from build123d import *

# Parameters (mm, degrees)
F0_R     = 3.175
F1_DEPTH = 3.175
F2_R     = 8.1915


with BuildPart() as f1:
    # F0 (on Top) → F1 (new body)
    with BuildSketch(Plane.XY):
        with BuildLine():
            ThreePointArc((-15.5081209619, -65.37452), (-10.36179917, -75.1896860078), (0, -79.121))
            ThreePointArc((0, -79.121), (10.36179917, -75.1896860078), (15.5081209619, -65.37452))
            ThreePointArc((15.5081209619, -65.37452), (15.5927547044, -64.4389577876), (15.621, -63.5))
            ThreePointArc((15.621, -63.5), (15.602952529, -62.7493247194), (15.5488518178, -62.000384))
            ThreePointArc((15.5488518178, -62.000384), (0, -47.879), (-15.5488518178, -62.000384))
            ThreePointArc((-15.5488518178, -62.000384), (-15.6198619711, -63.6885550396), (-15.5081209619, -65.37452))
        make_face()
        with BuildLine():
            ThreePointArc((0, -66.675), (-2.2450640303, -61.2549359697), (3.175, -63.5))
            ThreePointArc((3.175, -63.5), (2.2450640303, -65.7450640303), (0, -66.675))
        make_face(mode=Mode.SUBTRACT)
        with BuildLine():
            ThreePointArc((15.5081209619, -65.37452), (10.36179917, -75.1896860078), (0, -79.121))
            Line((0, -79.121), (0, -100.0125))
            Line((0, -100.0125), (0, -104.775))
            ThreePointArc((0, -104.775), (6.7351920908, -107.5648079092), (9.525, -114.3))
            ThreePointArc((9.525, -114.3), (9.5077772588, -114.8725352363), (9.4561713182, -115.443))
            Line((9.4561713182, -115.443), (15.5081209619, -65.37452))
        make_face()
        with BuildLine():
            ThreePointArc((6.35, -100.0125), (3.175, -103.1875), (0, -100.0125))
            ThreePointArc((0, -100.0125), (3.175, -96.8375), (6.35, -100.0125))
        make_face(mode=Mode.SUBTRACT)
        with BuildLine():
            Line((0, -100.0125), (0, -79.121))
            ThreePointArc((0, -79.121), (-10.36179917, -75.1896860078), (-15.5081209619, -65.37452))
            Line((-15.5081209619, -65.37452), (-9.4561713182, -115.443))
            ThreePointArc((-9.4561713182, -115.443), (-7.1278573218, -107.9818297744), (0, -104.775))
            Line((0, -104.775), (0, -100.0125))
        make_face()
        with BuildLine():
            ThreePointArc((9.525, -114.3), (6.7351920908, -107.5648079092), (0, -104.775))
            ThreePointArc((0, -104.775), (-7.1278573218, -107.9818297744), (-9.4561713182, -115.443))
            ThreePointArc((-9.4561713182, -115.443), (0, -123.825), (9.4561713182, -115.443))
            ThreePointArc((9.4561713182, -115.443), (9.5077772588, -114.8725352363), (9.525, -114.3))
        make_face()
        with BuildLine():
            ThreePointArc((3.175, -114.3), (-2.2450640303, -116.5450640303), (0, -111.125))
            ThreePointArc((0, -111.125), (2.2450640303, -112.0549359697), (3.175, -114.3))
        make_face(mode=Mode.SUBTRACT)
        with BuildLine():
            Line((-10.4524001899, -9.157542126), (-15.5488518178, -62.000384))
            ThreePointArc((-15.5488518178, -62.000384), (0, -47.879), (15.5488518178, -62.000384))
            Line((15.5488518178, -62.000384), (9.481007206, 0.9144))
            ThreePointArc((9.481007206, 0.9144), (9.5139954445, 0.4577288296), (9.525, 0))
            ThreePointArc((9.525, 0), (6.6138273175, -6.8544083052), (-0.3401786278, -9.5189234423))
            Line((-0.3401786278, -9.5189234423), (-10.4524001899, -9.157542126))
        make_face()
        with BuildLine():
            Line((-9.481007206, 0.9144), (-10.4524001899, -9.157542126))
            Line((-10.4524001899, -9.157542126), (-0.3401786278, -9.5189234423))
            ThreePointArc((-0.3401786278, -9.5189234423), (-7.164320087, -6.2767939819), (-9.481007206, 0.9144))
        make_face()
        with BuildLine():
            Line((-44.7334821429, -7.9324362036), (-10.4524001899, -9.157542126))
            Line((-10.4524001899, -9.157542126), (-9.481007206, 0.9144))
            ThreePointArc((-9.481007206, 0.9144), (-6.5286581491, 6.9355784022), (-0.3401783155, 9.5189234535))
            Line((-0.3401783155, 9.5189234535), (-44.7334821429, 7.9324362036))
            ThreePointArc((-44.7334821429, 7.9324362036), (-38.9384772185, 5.7120069047), (-36.5125, 0))
            ThreePointArc((-36.5125, 0), (-38.9384772185, -5.7120069047), (-44.7334821429, -7.9324362036))
        make_face()
        with BuildLine():
            ThreePointArc((9.525, 0), (9.5139954445, 0.4577288296), (9.481007206, 0.9144))
            ThreePointArc((9.481007206, 0.9144), (6.2767940994, 7.164319984), (-0.3401783155, 9.5189234535))
            ThreePointArc((-0.3401783155, 9.5189234535), (-6.5286581491, 6.9355784022), (-9.481007206, 0.9144))
            ThreePointArc((-9.481007206, 0.9144), (-7.164320087, -6.2767939819), (-0.3401786278, -9.5189234423))
            ThreePointArc((-0.3401786278, -9.5189234423), (6.6138273175, -6.8544083052), (9.525, 0))
        make_face()
        Circle(F0_R, mode=Mode.SUBTRACT)
        with BuildLine():
            ThreePointArc((-44.7334821429, 7.9324362036), (-52.3875, 0), (-44.7334821429, -7.9324362036))
            ThreePointArc((-44.7334821429, -7.9324362036), (-38.9384772185, -5.7120069047), (-36.5125, 0))
            ThreePointArc((-36.5125, 0), (-38.9384772185, 5.7120069047), (-44.7334821429, 7.9324362036))
        make_face()
        with Locations((-44.45, 0)):
            Circle(F0_R, mode=Mode.SUBTRACT)
    extrude(amount=F1_DEPTH)

    # F2
    f2_edges = [f1.edges().sort_by_distance(p)[0] for p in [
        (-10.4524, -9.157542, 1.5875),
    ]]
    fillet(f2_edges, radius=F2_R)


solid = f1.part
Can you work these out from the model? Positions are in its coordinate system, mm. A direction names the side the tool comes from. Give positions to 0.01 mm unless a question says otherwise; leave off trailing zeros. Loops run counter-clockwise (first coordinate to the right, second up) from the corner with the lowest first, then second, coordinate; pieces in that order, holes last. Notation, with made-up numbers: (-7, -11.5) - (29, -11.5) arc R19 ccw to (29, 21.5) - close; hole circle Ø1 at (73.5, -6.5). An arc over 180 degrees is marked (long way). One line per item, written item: value.
(1) If we section it at A-A, the plane x = -13.5: List the corners of the cut face in (y, z) for me (3 decimals).
Verdict:
outline: (-81.988, 0) - (-40.757, 0) - (-40.757, 3.175) - (-81.988, 3.175) - close; (-11.394, 0) - (9.049, 0) - (9.049, 3.175) - (-11.394, 3.175) - close
(2) I'm going to push flat-ended pins straight in: pin 1 (4 mm diameter, centred on x = 0, y = -63.5, fed in from +Z); pin 2 (1.5 mm diameter, centred on y = -10, z = 0.5, fed in from +X); pin 3 (7.5 mm diameter, centred on x = 0, y = -114.3, fed in from +Z) (3 decimals); pin 4 (1 mm diameter, centred on y = -37.5, z = 2, fed in from +X). Where does each tip first touch, or does it pass through?
Verdict:
pin 1: through
pin 2: x = 10.61
pin 3: z = 3.175
pin 4: x = 13.23
(3) If we mould it in two halves opening along X, with no side actions, what happens to faces 1 (the face through (12.557, -30.983, 1.565)), 2 (the face through (3.863, -103.112, 1.565)), 3 (the face through (-12.525, -90.058, 1.565)), 4 (the face through (-0.69, -3.1, 1.57))? For each: released by +X, released by -X, zero draft, split by the parting line, or undercut.
Verdict:
face 1: released by +X
face 2: undercut
face 3: released by -X
face 4: undercut
(4) On a 3-axis mill with a long thin cutter (end or side, diameter ignored), from which of +Z, -Z, +X, -X, +Y, -Y can I reach the whole of each face in a straight line? I mean faces 5 (the face through (-41.42, 0.95, 1.57)), 6 (the face through (-13.39, -39.6, 1.57)). Say none if no direction works.
Verdict:
face 5: +Z, -Z
face 6: +Z, -Z, -X
(5) If we section it at D-D, the plane y = -46: List the corners of the cut face in (x, z) for me (3 decimals).
Verdict:
outline: (-14.006, 0) - (14.006, 0) - (14.006, 3.175) - (-14.006, 3.175) - close
(6) I need wall thicknesses on line 1 along Y through (x, z) = (-44.45, 0.7) (3 decimals); line 2 along X through (y, z) = (-63.5, 0.9) (3 decimals); line 3 along Y through (x, z) = (-1.5, 0.7). Which ranges of each line are inside material? Lowest first, please.
Verdict:
line 1: -7.943 to -3.175, 3.175 to 7.943
line 2: -15.621 to -3.175, 3.175 to 15.621
line 3: -123.71 to -117.1, -111.5 to -66.3, -60.7 to -2.8, 2.8 to 9.48
(7) If we section it at C-C, the plane x = -43: List the corners of the cut face in (y, z) for me (3 decimals), plus the area to 3 significant figures.
Verdict:
outline: (-7.994, 0) - (-2.825, 0) - (-2.825, 3.175) - (-7.994, 3.175) - close; (2.825, 0) - (7.994, 0) - (7.994, 3.175) - (2.825, 3.175) - close
area: 32.8 mm^2
(8) If we section it at B-B, the plane z = 2.1: State how many separate pieces and enclosed holes the cut face has, plus the area to 3 significant figures.
Verdict:
separate pieces: 1
enclosed holes: 5
area: 3,740 mm^2
